Autodesk Inventor part; units mm, degrees
ref_plane "YZ Plane" through (0, 0, 0) normal (1, 0, 0) x (0, 1, 0)
ref_plane "XZ Plane" through (0, 0, 0) normal (0, 1, 0) x (-1, 0, 0)
ref_plane "XY Plane" through (0, 0, 0) normal (0, 0, 1) x (1, 0, 0)
sketch "Sketch1" plane through (0, 0, 0) normal (1, 0, 0) x (0, 1, 0)
  line L0 (0, 0) -> (0, -30) construction
  line L1 (-7.5, 0) -> (-7.5, -30)
  line L2 (7.5, -30) -> (7.5, 0)
  arc A0 (7.5, 0) -> (-7.5, 0) centre (0, 0) ccw
  arc A1 (-7.5, -30) -> (7.5, -30) centre (0, -30) ccw
  point P0 (0, -15)
  dimension "d0" = 7.5
  dimension "d1" = 30
extrude "Extrusion1" add sketch "Sketch1" against normal blind 10
sketch "Sketch2" plane through (0, 0, 0) normal (1, 0, 0) x (0, 0, -1)
  line L0 (37.5, -7.5) -> (15, -7.5)
  line L1 (15, -7.5) -> (15, 7.5)
  line L2 (15, 7.5) -> (37.5, 7.5)
  line L3 (37.5, 7.5) -> (37.5, -7.5)
  arc A0 (30, -7.5) -> (30, 7.5) centre (30, 0) ccw
  line L4 (0, -7.5) -> (30, -7.5)
  line L5 (30, 7.5) -> (0, 7.5)
  point P0 (0, 0)
  point P1 (37.5, 0)
  point P2 (26.25, -7.5)
  point P3 (26.25, 7.5)
  point P4 (30, 7.5)
  point P5 (30, -7.5)
  dimension "d4" = 22.5
extrude "Extrusion2" cut sketch "Sketch2" against normal blind 10 contours L0 L1 L2 A0
sketch "Sketch3" plane through (0, 0, 0) normal (1, 0, 0) x (0, 0, -1)
  circle A0 centre (0, 0) radius 3.2
  line L0 (15, -7.5) -> (15, 7.5)
  point P0 (0, 0)
  dimension "d7" = 6.4
  dimension "d17" = 15
  dimension "d18" = 16.7705
extrude "Extrusion3" cut sketch "Sketch3" against normal blind 10
sketch "Sketch4" plane through (0, 0, 0) normal (1, 0, 0) x (0, 0, -1)
  circle A0 centre (0, 0) radius 5.5
  dimension "d11" = 11
extrude "Extrusion4" cut sketch "Sketch4" against normal blind 6.8
sketch "Sketch5" plane through (0, 0, 0) normal (1, 0, 0) x (0, 0, -1)
  line L0 (15, -7.5) -> (15, 7.5)
  circle A0 centre (15, 0) radius 5
  point P0 (0, 0)
  point P1 (15, 5)
  point P2 (15, -5)
  dimension "d14" = 10
extrude "Extrusion5" cut sketch "Sketch5" against normal through all contours A0 L0 picked at (13.3455, -0.2009)
The listing builds one solid part. Answer for the finished solid, in the listing's coordinates (mm). A direction names the side the tool comes from. Coordinates: 2 decimals unless noted, no trailing zeros. Loops run counter-clockwise (first coordinate to the right, second up) from the corner with the lowest first, then second, coordinate; pieces in that order, holes last.
1) Flat-ended cylindrical pins translate along their axes: pin 1 Ø5 at (x, y) = (-5.5, 2) entering from -Z; pin 2 Ø4 at (y, z) = (0, 0) entering from -X. Find the tip coordinate at first contact, or state that the pin passes through.
2) Find section C-C on z = -2. Write down the section's boundary in (x, y).
3) Find section D-D on z = -5. Write down the section's boundary in (x, y).
4) Find the intervals of material crossed by L1, parallel to Y at x = -9.2, z = 0; L2, parallel to Y at x = -2.75, z = 0; L3, parallel to X at y = -1.75, z = -4.25, in increasing order.
5) Find section A-A on y = 0. Write down the section's boundary in (x, z).
6) Determine the mould class of faces 1 (the face through (-5, 7.5, -8)), 2 (the face through (0, 0, -6)), 3 (the face through (-6.8, -2.4, -2.4)) for opening direction Y: pulls with the +Y half, pulls with the -Y half, needs draft (parallel to the pull), parting line crosses it, or undercut.
7) A tool of negligible diameter and unlimited length cuts with its end or side. For faces 4 (the face through (-3.35, -5.37, 1.19)), 5 (the face through (-5, 0, -10)), from which of +Z, -Z, +X, -X, +Y, -Y can it reach the whole face along a straight path? Write none if from no direction.
8) Find section B-B on x = -3. Write down the section's boundary in (y, z).
Values:
1. pin 1: stops at z = -12.82
1. pin 2: passes through
2. outline: (-10, -7.5) - (0, -7.5) - (0, -5.12) - (-6.8, -5.12) - (-6.8, -2.5) - (-10, -2.5) - close; (-10, 2.5) - (-6.8, 2.5) - (-6.8, 5.12) - (0, 5.12) - (0, 7.5) - (-10, 7.5) - close
3. outline: (-10, -7.5) - (0, -7.5) - (0, -2.29) - (-6.8, -2.29) - (-6.8, 2.29) - (0, 2.29) - (0, 7.5) - (-10, 7.5) - close
4. L1: y = -7.5 to -3.2, 3.2 to 7.5
4. L2: y = -7.5 to -5.5, 5.5 to 7.5
4. L3: x = -10 to -6.8
5. outline: (-10, -10) - (0, -10) - (0, -5.5) - (-6.8, -5.5) - (-6.8, -3.2) - (-10, -3.2) - close; (-10, 3.2) - (-6.8, 3.2) - (-6.8, 5.5) - (0, 5.5) - (0, 7.5) - (-10, 7.5) - close
6. face 1: pulls with the +Y half
6. face 2: needs draft
6. face 3: undercut
7. face 4: +X
7. face 5: -Z, +X, -X
8. outline: (-7.5, -15) - (-5, -15) arc R5 cw to (5, -15) - (7.5, -15) - (7.5, 0) arc R7.5 ccw to (-7.5, 0) - close; hole circle Ø11 at (0, 0)
